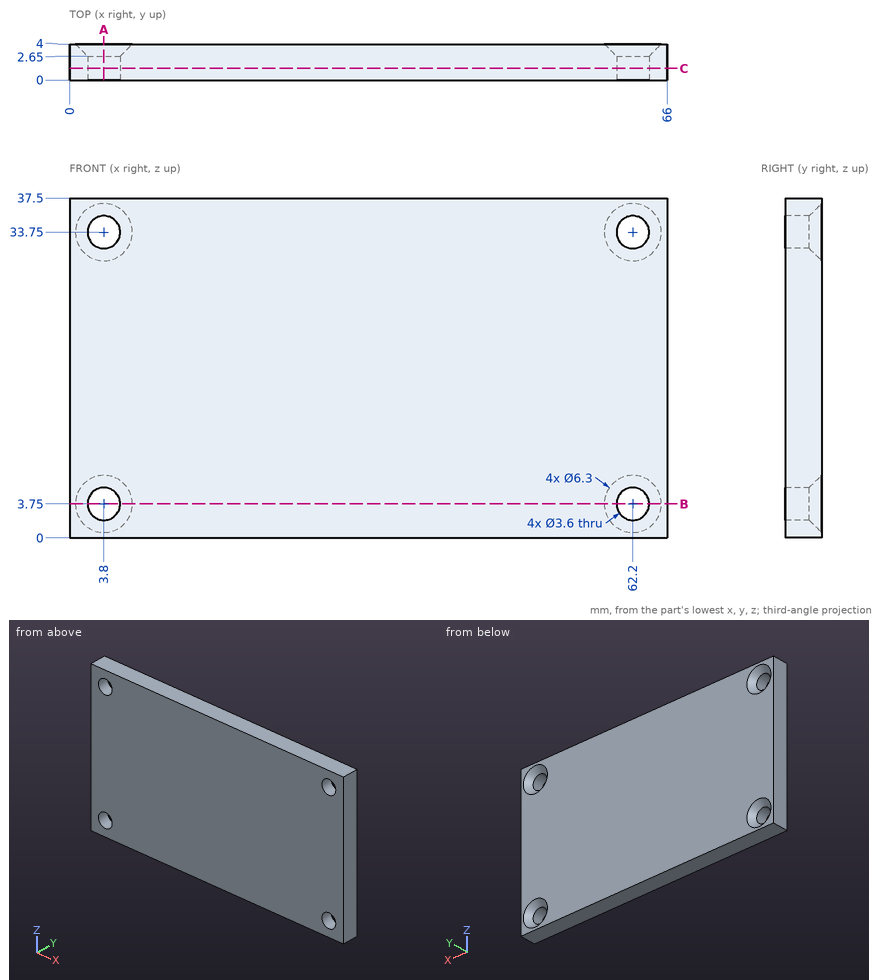
Could you check a few things on this drawing? It's one solid part, dimensions in mm from its lowest x, y, z. Coordinates: 2 decimals unless noted, no trailing zeros. Write each loop counter-clockwise with the first axis right and the second up, starting at its lowest first coordinate (ties: lowest second). Pieces come first, ordered by that corner, then holes. Notation, with made-up numbers: M 18,38.5 L 54,38.5 A12 ccw 54,45.5 Z; hole C 59,73 d1. An arc over 180 degrees is marked long. Answer as CSV lines item,"result". Start each with the question number.
Q1. Suppose I cut it at A-A, the plane x = 3.8. List the corners of the cut face in (y, z) for me.
Q2. Will this pin go through, and if not, where does the flat tip stop? pin 1 Ø2 at (x, z) = (62.2, 33.75) entering from -Y.
Q3. Suppose I cut it at B-B, the plane z = 3.75. List the corners of the cut face in (x, y) for me, then the cut area to 3 significant figures.
Q4. Suppose I cut it at C-C, the plane y = 1.3. List the corners of the cut face in (x, z) for me.
Q5. I need wall thicknesses on probe 1 along Z at (x, y) = (62.2, 1.9); probe 2 along X at (y, z) = (0.7, 3.75); probe 3 along Z at (x, y) = (5, 1.2). Which ranges of each line are inside material? Lowest first, please. Write a range as [from, to].
Entries:
1,outline,"M 0,0 L 4,0 L 4,0.6 L 2.65,1.95 L 0,1.95 Z; M 0,5.55 L 2.65,5.55 L 4,6.9 L 4,30.6 L 2.65,31.95 L 0,31.95 Z; M 0,35.55 L 2.65,35.55 L 4,36.9 L 4,37.5 L 0,37.5 Z"
2,pin 1,"passes through"
3,outline,"M 0,0 L 2,0 L 2,2.65 L 0.65,4 L 0,4 Z; M 5.6,0 L 60.4,0 L 60.4,2.65 L 59.05,4 L 6.95,4 L 5.6,2.65 Z; M 64,0 L 66,0 L 66,4 L 65.35,4 L 64,2.65 Z"
3,area,"232 mm²"
4,outline,"M 0,0 L 66,0 L 66,37.5 L 0,37.5 Z; hole C 3.8,3.75 d3.6; hole C 3.8,33.75 d3.6; hole C 62.2,3.75 d3.6; hole C 62.2,33.75 d3.6"
5,probe 1,"z = [0, 1.95], [5.55, 31.95], [35.55, 37.5]"
5,probe 2,"x = [0, 2], [5.6, 60.4], [64, 66]"
5,probe 3,"z = [0, 2.41], [5.09, 32.41], [35.09, 37.5]"
